Geometry: final body of the model. Coordinates: model frame, mm. Face numbers are marked on the shaded views. Give positions to 0.01 mm unless a question says otherwise; leave off trailing zeros. Write each loop counter-clockwise with the first axis right and the second up, starting at its lowest first coordinate (ties: lowest second). Pieces come first, ordered by that corner, then holes. Notation, with made-up numbers: (46, 58.25) - (83, 58.25) arc R14 cw to (83, 82.25) - close; hole circle Ø1 at (63, 76). An arc over 180 degrees is marked (long way). Return JSON: item names as keys, results as strings.
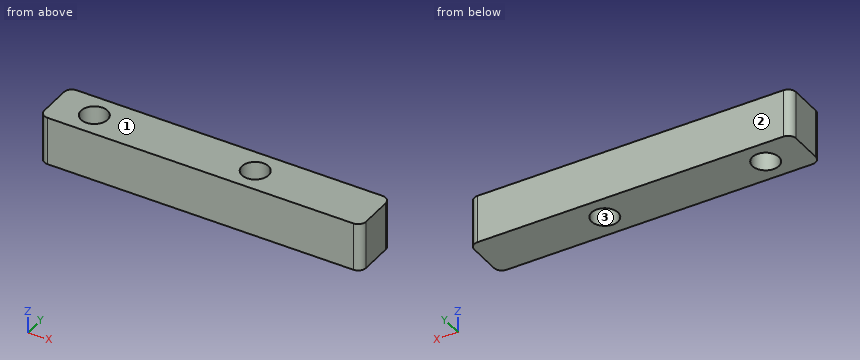
from build123d import *

# Parameters (mm, degrees)
SKETCH_1_W          = 40
SKETCH_1_H          = 6
EXTRUDE_1_DEPTH     = 6
SKETCH_2_R          = 1.65
CUT_EXTRUDE_1_DEPTH = 6
FILLET_1_R          = 1


with BuildPart() as part:
    # 草图1 → 凸台-拉伸1 (new body)
    with BuildSketch(Plane.XY):
        Rectangle(SKETCH_1_W, SKETCH_1_H)
    extrude(amount=EXTRUDE_1_DEPTH)

    # 草图2 → 切除-拉伸1 (cut)
    with BuildSketch(Plane.XY.offset(6)):
        with Locations((5, 0)):
            Circle(SKETCH_2_R)
        with Locations((-15, 0)):
            Circle(SKETCH_2_R)
    extrude(amount=-CUT_EXTRUDE_1_DEPTH, mode=Mode.SUBTRACT)

    # 圆角1
    fillet_1_edges = [part.edges().sort_by_distance(p)[0] for p in [
        (20, -3, 3),
        (-20, -3, 3),
        (-20, 3, 3),
        (20, 3, 3),
    ]]
    fillet(fillet_1_edges, radius=FILLET_1_R)


solid = part.part
Q1. Mould query, pull axis Y, two halves, no side actions, for the marked faces 1, 2 and 3. Classes: pulls with the +Y half, pulls with the -Y half, needs draft (parallel to the pull), parting line crosses it, or undercut.
Answer key:
{"face 1": "needs draft", "face 2": "pulls with the +Y half", "face 3": "undercut"}
Q2. Section query B-B, the plane y = 0. Return the cut outline in (x, z).
Answer key:
{"outline": "(-20, 0) - (-16.65, 0) - (-16.65, 6) - (-20, 6) - close; (-13.35, 0) - (3.35, 0) - (3.35, 6) - (-13.35, 6) - close; (6.65, 0) - (20, 0) - (20, 6) - (6.65, 6) - close"}
Q3. Section query C-C, the plane x = 5. Return the cut outline in (y, z), plus the area to 3 significant figures.
Answer key:
{"outline": "(-3, 0) - (-1.65, 0) - (-1.65, 6) - (-3, 6) - close; (1.65, 0) - (3, 0) - (3, 6) - (1.65, 6) - close", "area": "16.2 mm^2"}
Q4. Material intervals for probe 1 along X at (y, z) = (0.05, 2.9); probe 2 along Y at (x, z) = (-15, 1.5); probe 3 along X at (y, z) = (-0.65, 1.1), sorted ascending. Write a range as [from, to].
Answer key:
{"probe 1": "x = [-20, -16.65], [-13.35, 3.35], [6.65, 20]", "probe 2": "y = [-3, -1.65], [1.65, 3]", "probe 3": "x = [-20, -16.52], [-13.48, 3.48], [6.52, 20]"}
Q5. Pin query (flat end, axial travel): P1, Ø3, axis at x = 5, y = 0, coming from the +Z side. Return the tip coordinate at first contact, or that it passes through.
Answer key:
{"P1": "passes through"}
Q6. Section query A-A, the plane z = 4.5. Return the cut outline in (x, y), plus the area to 3 significant figures.
Answer key:
{"outline": "(-20, -2) arc R1 ccw to (-19, -3) - (19, -3) arc R1 ccw to (20, -2) - (20, 2) arc R1 ccw to (19, 3) - (-19, 3) arc R1 ccw to (-20, 2) - close; hole circle Ø3.3 at (-15, 0); hole circle Ø3.3 at (5, 0)", "area": "222 mm^2"}
